Input: part model. Units: mm. Frame: model coordinates. A direction names the side the tool comes from. Give positions to 0.01 mm unless a question says otherwise; leave off trailing zeros. Write each loop counter-clockwise with the first axis right and the second up, starting at its lowest first coordinate (ties: lowest second). Pieces come first, ordered by that corner, then holes. Notation, with made-up numbers: (10.25, -32.5) - (52.25, -32.5) arc R22 cw to (52.25, -24.5) - close; hole circle Ø8 at (73, 66.25). An arc over 180 degrees is marked (long way). Answer as a JSON object with one key per item and string values. Group by question number.
from build123d import *

# Parameters (mm, degrees)
SKETCH1_W                 = 51
SKETCH1_H                 = 10
SKETCH1_R                 = 2.55
BOSS_EXTRUDE1_DEPTH       = 5
SKETCH3_W                 = 10
SKETCH3_H                 = 25
SKETCH3_W_2               = 6
SKETCH3_H_2               = 21
BOSS_EXTRUDE2_DEPTH       = 5
SKETCH5_W                 = 25
SKETCH5_H                 = 24
BOSS_EXTRUDE3_DEPTH       = 5
FILLET1_R                 = 20
SKETCH6_R                 = 1.75
BOSS_EXTRUDE4_DEPTH       = 3
CHAMFER1_SIZE             = 3
M2X0_4_TAPPED_HOLE1_D     = 1.6
M2X0_4_TAPPED_HOLE1_DEPTH = 9.2
M2X0_4_TAPPED_HOLE1_TIP   = 0.480688495
FILLET2_R                 = 2


with BuildPart() as part:
    # Sketch1 → Boss-Extrude1 (new body)
    with BuildSketch(Plane.XY):
        with Locations((25.5, 5)):
            Rectangle(SKETCH1_W, SKETCH1_H)
        with Locations((5, 5)):
            Circle(SKETCH1_R, mode=Mode.SUBTRACT)
        with Locations((46, 5)):
            Circle(SKETCH1_R, mode=Mode.SUBTRACT)
    extrude(amount=BOSS_EXTRUDE1_DEPTH)

    # Sketch3 → Boss-Extrude2 (add)
    with BuildSketch(Plane.XY.offset(5)):
        with Locations((-5, -2.5)):
            Rectangle(SKETCH3_W, SKETCH3_H)
        with Locations((-5, -2.5)):
            Rectangle(SKETCH3_W_2, SKETCH3_H_2, mode=Mode.SUBTRACT)
    extrude(amount=-BOSS_EXTRUDE2_DEPTH)

    # Sketch5 → Boss-Extrude3 (add)
    with BuildSketch(Plane(origin=(51, 0, 0), x_dir=(0, 0, -1), z_dir=(1, 0, 0))):
        with Locations((-12.5, -12)):
            Rectangle(SKETCH5_W, SKETCH5_H)
    extrude(amount=-BOSS_EXTRUDE3_DEPTH)

    # Fillet1
    fillet1_edges = [part.edges().sort_by_distance(p)[0] for p in [
        (46, 0, 2.5),
    ]]
    fillet(fillet1_edges, radius=FILLET1_R)

    # Sketch6 → Boss-Extrude4 (add)
    with BuildSketch(Plane(origin=(51, 0, 0), x_dir=(0, 0, -1), z_dir=(1, 0, 0))):
        with Locations(Location((-23, -9.5, 0), (0, 0, 180))):
            Circle(SKETCH6_R)
        with Locations(Location((-23, -22, 0), (0, 0, 180))):
            Circle(SKETCH6_R)
        with Locations(Location((-2, -22, 0), (0, 0, 180))):
            Circle(SKETCH6_R)
        with Locations(Location((-2, -9.5, 0), (0, 0, 180))):
            Circle(SKETCH6_R)
    extrude(amount=BOSS_EXTRUDE4_DEPTH)

    # Chamfer1
    # the kernel refuses this chamfer: 3 mm, written as the material it adds along each edge
    with BuildSketch(Plane(origin=(51, -9.5, 23), x_dir=(0, 0, 1), z_dir=(0, 1, 0))) as chamfer1_piece_1_section:
        Polygon((1.75 + CHAMFER1_SIZE, 0), (1.75, CHAMFER1_SIZE), (1.75, 0), align=None)
    chamfer1_piece_1 = revolve(axis=Axis((51, -9.5, 23), (1, 0, 0)), mode=Mode.PRIVATE)
    chamfer1_piece_1 = split(chamfer1_piece_1, bisect_by=Plane(origin=(52.428955804, -9.5, 25), z_dir=(0, 0, -1)), keep=Keep.TOP, mode=Mode.PRIVATE)
    chamfer1_piece_1 = split(chamfer1_piece_1, bisect_by=Plane(origin=(54, -9.5, 19.736191383), z_dir=(-1, 0, 0)), keep=Keep.TOP, mode=Mode.PRIVATE)
    add(chamfer1_piece_1)
    with BuildSketch(Plane(origin=(51, -22, 23), x_dir=(0, 0, 1), z_dir=(0, 1, 0))) as chamfer1_piece_2_section:
        Polygon((1.75 + CHAMFER1_SIZE, 0), (1.75, CHAMFER1_SIZE), (1.75, 0), align=None)
    chamfer1_piece_2 = revolve(axis=Axis((51, -22, 23), (1, 0, 0)), mode=Mode.PRIVATE)
    chamfer1_piece_2 = split(chamfer1_piece_2, bisect_by=Plane(origin=(52.431534605, -24, 19.733612581), z_dir=(0, 1, 0)), keep=Keep.TOP, mode=Mode.PRIVATE)
    chamfer1_piece_2 = split(chamfer1_piece_2, bisect_by=Plane(origin=(52.431534605, -22, 25), z_dir=(0, 0, -1)), keep=Keep.TOP, mode=Mode.PRIVATE)
    chamfer1_piece_2 = split(chamfer1_piece_2, bisect_by=Plane(origin=(54, -22, 19.733612581), z_dir=(-1, 0, 0)), keep=Keep.TOP, mode=Mode.PRIVATE)
    add(chamfer1_piece_2)
    with BuildSketch(Plane(origin=(51, -22, 2), x_dir=(0, 0, 1), z_dir=(0, 1, 0))) as chamfer1_piece_3_section:
        Polygon((1.75 + CHAMFER1_SIZE, 0), (1.75, CHAMFER1_SIZE), (1.75, 0), align=None)
    chamfer1_piece_3 = revolve(axis=Axis((51, -22, 2), (1, 0, 0)), mode=Mode.PRIVATE)
    chamfer1_piece_3 = split(chamfer1_piece_3, bisect_by=Plane(origin=(53.459818879, -23.938254184, 0), z_dir=(0, 0, 1)), keep=Keep.TOP, mode=Mode.PRIVATE)
    chamfer1_piece_3 = split(chamfer1_piece_3, bisect_by=Plane(origin=(53.459818879, -24, 3.119051575), z_dir=(0, 1, 0)), keep=Keep.TOP, mode=Mode.PRIVATE)
    chamfer1_piece_3 = split(chamfer1_piece_3, bisect_by=Plane(origin=(54, -23.938254184, 3.119051575), z_dir=(-1, 0, 0)), keep=Keep.TOP, mode=Mode.PRIVATE)
    add(chamfer1_piece_3)
    with BuildSketch(Plane(origin=(51, -9.5, 2), x_dir=(0, 0, 1), z_dir=(0, 1, 0))) as chamfer1_piece_4_section:
        Polygon((1.75 + CHAMFER1_SIZE, 0), (1.75, CHAMFER1_SIZE), (1.75, 0), align=None)
    chamfer1_piece_4 = revolve(axis=Axis((51, -9.5, 2), (1, 0, 0)), mode=Mode.PRIVATE)
    chamfer1_piece_4 = split(chamfer1_piece_4, bisect_by=Plane(origin=(51.400671534, -13.217061478, 0), z_dir=(0, 0, 1)), keep=Keep.TOP, mode=Mode.PRIVATE)
    chamfer1_piece_4 = split(chamfer1_piece_4, bisect_by=Plane(origin=(54, -13.217061478, 4.146046445), z_dir=(-1, 0, 0)), keep=Keep.TOP, mode=Mode.PRIVATE)
    add(chamfer1_piece_4)

    # M2x0.4 Tapped Hole1
    with Locations(Plane(origin=(54, 0, 0), x_dir=(0, 0, -1), z_dir=(1, 0, 0))):
        with Locations((-23, -22), (-23, -9.5), (-2, -9.5), (-2, -22)):
            Hole(M2X0_4_TAPPED_HOLE1_D / 2, depth=M2X0_4_TAPPED_HOLE1_DEPTH)
            with Locations((0, 0, -(M2X0_4_TAPPED_HOLE1_DEPTH + M2X0_4_TAPPED_HOLE1_TIP / 2))):  # 118° drill point
                Cone(0, M2X0_4_TAPPED_HOLE1_D / 2, M2X0_4_TAPPED_HOLE1_TIP, mode=Mode.SUBTRACT)

    # Fillet2
    fillet2_edges = [part.edges().sort_by_distance(p)[0] for p in [
        (0, -15, 2.5),
        (-10, -15, 2.5),
        (-10, 10, 2.5),
        (-2, -13, 2.5),
        (-8, -13, 2.5),
        (-8, 8, 2.5),
        (-2, 8, 2.5),
        (0, 0, 2.5),
    ]]
    fillet(fillet2_edges, radius=FILLET2_R)


solid = part.part
1) Reachability of faces 1 (the face through (40.297, -6.014, 2.465)), 2 (the face through (-8, -3, 3)), 3 (the face through (49, -24, 12)) from +Z, -Z, +X, -X, +Y, -Y: full face, straight path, thin tool, end or side. Return the list, or none.
2) Cut plane A-A on y = -22. Return the cut outline in (x, z).
3) Cut plane D-D on y = -1. Return the cut outline in (x, z) (3 decimals), and give its area (3 significant figures).
4) Mould query, pull axis Z, two halves, no side actions, for faces 4 (the face through (53.854, -9.583, 21.106)), 5 (the face through (0.57, -0.6, 2.54)), 6 (the face through (29, 1, 0)). Classes: +Z half, -Z half, draft (parallel to the pull), parting line (faces both ways), or undercut.
5) Pin query (flat end, axial travel): P1, Ø6, axis at y = -15.5, z = 14.5, coming from the +X side; P2, Ø4, axis at y = -2, z = 22, coming from the -X side; P3, Ø1.5, axis at x = 49, z = 17.5, coming from the +Y side. Return the tip coordinate at first contact, or that it passes through.
6) Cut plane B-B on x = 5. Return the cut outline in (y, z), and give its area (3 significant figures).
7) Line query: line 1 along Y through (x, z) = (48, 23); line 2 along Y through (x, z) = (49.5, 2); line 3 along Y through (x, z) = (5, 2.35). Output: solid intervals per line, ascending. Write a range as from..to.
8) Cut plane C-C on y = 5. Return the cut outline in (x, z), and give its area (3 significant figures).
Filled in:
{
 "1": {"face 1": "+Z, -Z, -Y", "face 2": "+Z, -Z", "face 3": "+Z, -Z, +X, -X, -Y"},
 "2": {"outline": "(46, 0) - (53.75, 0) - (54, 0.25) - (54, 1.2) - (46, 1.2) - close; (46, 2.8) - (54, 2.8) - (54, 3.75) - (51, 6.75) - (51, 18.25) - (54, 21.25) - (54, 22.2) - (46, 22.2) - close; (46, 23.8) - (54, 23.8) - (54, 24.75) - (53.75, 25) - (46, 25) - close"},
 "3": {"outline": "(-10, 0) - (-8, 0) - (-8, 5) - (-10, 5) - close; (-2, 0) - (0.268, 0) - (0.268, 5) - (-2, 5) - close; (32.245, 0) - (51, 0) - (51, 25) - (46, 25) - (46, 5) - (32.245, 5) - close", "area": "215 mm²"},
 "4": {"face 4": "undercut", "face 5": "draft", "face 6": "-Z half"},
 "5": {"P1": "stops at x = 51", "P2": "stops at x = 46", "P3": "stops at y = 0"},
 "6": {"outline": "(0, 0) - (2.45, 0) - (2.45, 5) - (0, 5) - close; (7.55, 0) - (10, 0) - (10, 5) - (7.55, 5) - close", "area": "24.5 mm²"},
 "7": {"line 1": "y = -24..-22.8, -21.2..-10.3, -8.7..0", "line 2": "y = -24..-22.8, -21.2..-10.3, -8.7..10", "line 3": "y = 0..2.45, 7.55..10"},
 "8": {"outline": "(-10, 0) - (-8, 0) - (-8, 5) - (-10, 5) - close; (-2, 0) - (2.45, 0) - (2.45, 5) - (-2, 5) - close; (7.55, 0) - (43.45, 0) - (43.45, 5) - (7.55, 5) - close; (48.55, 0) - (51, 0) - (51, 5) - (48.55, 5) - close", "area": "224 mm²"}
}
